```python
from build123d import *

# Parameters (mm, degrees)
SKETCH1_R           = 1.5
SKETCH1_W           = 41
SKETCH1_H           = 21
BOSS_EXTRUDE1_DEPTH = 3.5
SKETCH2_R           = 1.55
SKETCH2_W           = 3.5
SKETCH2_H           = 6
CUT_EXTRUDE1_DEPTH  = 63.723600024
SKETCH3_W           = 15
SKETCH3_H           = 3.5
CUT_EXTRUDE2_DEPTH  = 63.723600024
SKETCH4_R           = 1.5
CUT_EXTRUDE3_DEPTH  = 63.723600024
CUT_EXTRUDE5_REACH  = 64.724
SKETCH5_R           = 1.5


with BuildPart() as part:
    # Sketch1 → Boss-Extrude1 (new body)
    with BuildSketch(Plane.XY):
        with BuildLine():
            Line((-36, -31), (36, -31))
            ThreePointArc((36, -31), (38.121320344, -30.121320344), (39, -28))
            Line((39, -28), (39, 28))
            ThreePointArc((39, 28), (38.896468429, 28.781326206), (38.593019574, 29.508724458))
            Line((38.593019574, 29.508724458), (28.409114334, 47.011632611))
            ThreePointArc((28.409114334, 47.011632611), (26.428070455, 48.717592284), (23.81637841, 48.835481746))
            Line((23.81637841, 48.835481746), (-36.851532369, 30.876611309))
            ThreePointArc((-36.851532369, 30.876611309), (-38.403601164, 29.795188415), (-39, 28))
            Line((-39, 28), (-39, -28))
            ThreePointArc((-39, -28), (-38.121320344, -30.121320344), (-36, -31))
        make_face()
        with Locations((24.951754903, 45)):
            Circle(SKETCH1_R, mode=Mode.SUBTRACT)
        with Locations((-9.5, 14.5)):
            Rectangle(SKETCH1_W, SKETCH1_H, mode=Mode.SUBTRACT)
    extrude(amount=BOSS_EXTRUDE1_DEPTH)

    # Sketch2 → Cut-Extrude1 (cut, through all)
    with BuildSketch(Plane(origin=(0, 0, 0), x_dir=(-1, 0, 0), z_dir=(0, 0, -1))):
        with Locations((-34, -19.5)):
            Circle(SKETCH2_R)
        with Locations(Location((34, -19.5, 0), (0, 0, 180))):
            Circle(SKETCH2_R)
        with Locations((-34, -13)):
            Rectangle(SKETCH2_W, SKETCH2_H)
        with Locations((-34, -26)):
            Rectangle(SKETCH2_W, SKETCH2_H)
        with Locations((34, -26)):
            Rectangle(SKETCH2_W, SKETCH2_H)
        with Locations((34, -13)):
            Rectangle(SKETCH2_W, SKETCH2_H)
    extrude(amount=-CUT_EXTRUDE1_DEPTH, mode=Mode.SUBTRACT)

    # Sketch3 → Cut-Extrude2 (cut, through all)
    with BuildSketch(Plane(origin=(0, 0, 0), x_dir=(-1, 0, 0), z_dir=(0, 0, -1))):
        with Locations((19.75, -24.75)):
            Rectangle(SKETCH3_W, SKETCH3_H)
        with Locations((-19.75, -24.75)):
            Rectangle(SKETCH3_W, SKETCH3_H)
    extrude(amount=-CUT_EXTRUDE2_DEPTH, mode=Mode.SUBTRACT)

    # Sketch4 → Cut-Extrude3 (cut, through all)
    with BuildSketch(Plane(origin=(0, 0, 0), x_dir=(-1, 0, 0), z_dir=(0, 0, -1))):
        with Locations((-15, 19.25)):
            Circle(SKETCH4_R)
        with Locations((-15, 9.75)):
            Circle(SKETCH4_R)
        with Locations((34, 9.75)):
            Circle(SKETCH4_R)
        with Locations((34, 19.25)):
            Circle(SKETCH4_R)
    extrude(amount=-CUT_EXTRUDE3_DEPTH, mode=Mode.SUBTRACT)

    # Sketch5 → Cut-Extrude5 (cut, up to next)
    with BuildSketch(Plane(origin=(0, 0, 0), x_dir=(-1, 0, 0), z_dir=(0, 0, -1)), mode=Mode.PRIVATE) as cut_extrude5_sk1:
        with Locations((34, 0.25)):
            Circle(SKETCH5_R)
    cut_extrude5_tool1 = extrude(cut_extrude5_sk1.sketch, amount=-CUT_EXTRUDE5_REACH, mode=Mode.PRIVATE) & part.part
    add(cut_extrude5_tool1.solids().sort_by_distance((-34, 0.25, 0))[0], mode=Mode.SUBTRACT)


solid = part.part
```
For this review, take the finished solid that the model builds, in its own axes (mm). A direction names the side the tool comes from. Coordinates: 2 decimals unless noted, no trailing zeros. Write each loop counter-clockwise with the first axis right and the second up, starting at its lowest first coordinate (ties: lowest second). Pieces come first, ordered by that corner, then holes.
(1) Add section A-A on y = 19.25. Give the boundary of the cut face in (x, z).
(2) Add section D-D on x = 34. Give the boundary of the cut face in (y, z), then the cut area to 3 significant figures.
(3) The part is to be moulded in two halves that separate along Y. For faces 1 (the face through (26.463, 48.704, 1.726)), 2 (the face through (8, 1, 0)), 3 (the face through (-35.75, -26, 2)), say which applies: +Y half, -Y half, draft (parallel to the pull), parting line (faces both ways), or undercut.
(4) Add section B-B on y = -14.5. Give the boundary of the cut face in (x, z), then the cut area to 4 significant figures.
(5) Tool access review of faces 4 (the face through (-34, -16, 2)), 5 (the face through (-6.093, 39.982, 1.726)): name each direction out of +Z, -Z, +X, -X, +Y, -Y from which nothing blocks a thin tool from reaching the whole face with its end or side.
(6) Add section C-C on x = 9. Give the boundary of the cut face in (y, z).
(7) For pin 1 Ø1.5 at (x, z) = (21.5, 1) entering from +Y, flat-tipped, find the tip position at first contact; note if it passes through.
(8) Wall thickness on probe 1 along X at (y, z) = (-11, 1.5); probe 2 along Y at (x, z) = (-14.5, 2.6); probe 3 along Y at (x, z) = (-14, 1.55): over which ranges is each line inside the solid? List them lowest first.
Answer sheet:
1. outline: (-39, 0) - (-35.5, 0) - (-35.5, 3.5) - (-39, 3.5) - close; (-32.5, 0) - (-30, 0) - (-30, 3.5) - (-32.5, 3.5) - close; (11, 0) - (13.5, 0) - (13.5, 3.5) - (11, 3.5) - close; (16.5, 0) - (39, 0) - (39, 3.5) - (16.5, 3.5) - close
2. outline: (-31, 0) - (-29, 0) - (-29, 3.5) - (-31, 3.5) - close; (-23, 0) - (-21.05, 0) - (-21.05, 3.5) - (-23, 3.5) - close; (-17.95, 0) - (-16, 0) - (-16, 3.5) - (-17.95, 3.5) - close; (-10, 0) - (37.4, 0) - (37.4, 3.5) - (-10, 3.5) - close
2. area: 187 mm2
3. face 1: +Y half
3. face 2: draft
3. face 3: undercut
4. outline: (-39, 0) - (-35.75, 0) - (-35.75, 3.5) - (-39, 3.5) - close; (-32.25, 0) - (32.25, 0) - (32.25, 3.5) - (-32.25, 3.5) - close; (35.75, 0) - (39, 0) - (39, 3.5) - (35.75, 3.5) - close
4. area: 248.5 mm2
5. face 4: +Z, -Z
5. face 5: +Z, -Z, -X, +Y
6. outline: (-31, 0) - (4, 0) - (4, 3.5) - (-31, 3.5) - close; (25, 0) - (44.45, 0) - (44.45, 3.5) - (25, 3.5) - close
7. pin 1: stops at y = 48.37
8. probe 1: x = -39 to -35.75, -32.25 to 32.25, 35.75 to 39
8. probe 2: y = -31 to -26.5, -23 to 4, 25 to 37.49
8. probe 3: y = -31 to -26.5, -23 to 4, 25 to 37.64
